Autodesk Inventor part; units mm, degrees
ref_plane "YZ Plane" through (0, 0, 0) normal (1, 0, 0) x (0, 1, 0)
ref_plane "XZ Plane" through (0, 0, 0) normal (0, 1, 0) x (-1, 0, 0)
ref_plane "XY Plane" through (0, 0, 0) normal (0, 0, 1) x (1, 0, 0)
sketch "Sketch1" plane through (0, 0, 0) normal (0, 1, 0) x (-1, 0, 0)
  circle A0 centre (0, 0) radius 17.907
  dimension "d0" = 35.814
extrude "Extrusion1" add sketch "Sketch1" along normal blind 3.0734
sketch "Sketch2" plane through (0, 3.0734, 0) normal (0, 1, 0) x (1, 0, 0)
  circle A0 centre (0, 0) radius 8.001
  dimension "d3" = 16.002
extrude "Extrusion2" add sketch "Sketch2" along normal blind 1.397
fillet "Fillet1" radius 0.508 1 edges at (-8.001, 4.4704, 0)
fillet "Fillet2" radius 0.508 1 edges at (17.907, 3.0734, 0)
properties part number "speaker"
Design review of the part built by this model. Coordinates are the model's own, in mm. A direction names the side the tool comes from. Round coordinates to 2 decimals unless told otherwise and drop trailing zeros. Loops run counter-clockwise (first coordinate to the right, second up) from the corner with the lowest first, then second, coordinate; pieces in that order, holes last. Notation, with made-up numbers: (60.25, 62.5) - (96.25, 62.5) arc R27 ccw to (96.25, 93.5) - close; hole circle Ø9 at (45, 5.5). An arc over 180 degrees is marked (long way). One line per item, written item: value. Start each with the question number.
1) For faces 3 (the flat face through (0, 0, 0)), 4 (the cylindrical face through (-1.73, 3.51, -7.81)), list the 3-axis set-ups (+Z, -Z, +X, -X, +Y, -Y) from which the entire face can be reached by the end or side of a thin tool; tool diameter is ignored.
2) Insertion check: pin 1 Ø1.5 at (y, z) = (0.5, 12.5) entering from -X; pin 2 Ø10 at (x, z) = (7.5, 14) entering from +Y; pin 3 Ø1 at (y, z) = (2.5, -1.5) entering from +X. Each pin has a flat end and moves straight along its axis. Give the tip position at first contact, or say it passes through.
3) Consider section C-C on y = 1.4. Give the boundary of the cut face in (x, z), then the cut area to 3 significant figures.
4) To check wall thickness, follow L1, parallel to Y at x = 7, z = -14.5; L2, parallel to Z at x = 11, y = 1.5; L3, parallel to X at y = 1.25, z = -3.5. State the ranges of each line that lie inside material, in increasing order. Write a range as from..to.
5) Consider section A-A on z = 0. Give the boundary of the cut face in (x, y).
6) Draft analysis for pull direction Z (two halves, no side actions). For faces 1 (the flat face through (0, 4.47, 0)), 2 (the cylindrical face through (3.88, 1.26, 17.48)), state which applies: +Z half, -Z half, draft (parallel to the pull), parting line (faces both ways), or undercut.
7) Consider section B-B on x = 0. Give the boundary of the cut face in (y, z).
Reported:
1. face 3: +Z, -Z, +X, -X, -Y
1. face 4: +Y
2. pin 1: stops at x = -13.51
2. pin 2: stops at y = 3.07
2. pin 3: stops at x = 17.88
3. outline: circle Ø35.81 at (0, 0)
3. area: 1,010 mm^2
4. L1: y = 0..3.07
4. L2: z = -14.13..14.13
4. L3: x = -17.56..17.56
5. outline: (-17.91, 0) - (17.91, 0) - (17.91, 2.57) arc R0.51 ccw to (17.4, 3.07) - (8, 3.07) - (8, 3.96) arc R0.51 ccw to (7.49, 4.47) - (-7.49, 4.47) arc R0.51 ccw to (-8, 3.96) - (-8, 3.07) - (-17.4, 3.07) arc R0.51 ccw to (-17.91, 2.57) - close
6. face 1: draft
6. face 2: parting line
7. outline: (0, -17.91) - (2.57, -17.91) arc R0.51 ccw to (3.07, -17.4) - (3.07, -8) - (3.96, -8) arc R0.51 ccw to (4.47, -7.49) - (4.47, 7.49) arc R0.51 ccw to (3.96, 8) - (3.07, 8) - (3.07, 17.4) arc R0.51 ccw to (2.57, 17.91) - (0, 17.91) - close
